CAD build for the part. Positions are in the model's coordinates, mm. A direction names the side the tool comes from. Round coordinates to 2 decimals unless told otherwise and drop trailing zeros. Order: outer loops, then holes, each group sorted by start corner. A loop starts at its lowest first (then second) coordinate and runs counter-clockwise, first axis right, second up. Notation, with made-up numbers: M 42,81.25 L 54,81.25 A20 cw 54,94.25 Z; hole C 62.25,75.5 d6. An arc over 180 degrees is marked long. Answer as a JSON object with one key per item and string values. Group by question number.
Autodesk Inventor part; units mm, degrees
ref_plane "YZ Plane" through (0, 0, 0) normal (1, 0, 0) x (0, 1, 0)
ref_plane "XZ Plane" through (0, 0, 0) normal (0, 1, 0) x (-1, 0, 0)
ref_plane "XY Plane" through (0, 0, 0) normal (0, 0, 1) x (1, 0, 0)
sketch "Sketch1" plane through (0, 0, 0) normal (0, 0, 1) x (1, 0, 0)
  line L0 (0, 4) -> (0, -4)
  line L1 (0, -4) -> (1.25, -4)
  line L2 (1.25, -4) -> (1.5, -3.75)
  line L3 (1.5, -3.75) -> (1.5, 0.9)
  line L4 (1.6, 1) -> (2.5, 1)
  line L5 (2.75, 1.25) -> (2.75, 3.75)
  line L6 (2.5, 4) -> (0, 4)
  arc A0 (1.6, 1) -> (1.5, 0.9) centre (1.6, 0.9) ccw
  line L7 (2.5, 4) -> (2.75, 3.75)
  line L8 (2.5, 1) -> (2.75, 1.25)
  point P0 (0, 0)
  point P1 (2.75, 1)
  point P2 (2.75, 4)
  point P3 (0, 0)
  dimension "d0" = 5.5
  dimension "d1" = 3
  dimension "d3" = 3
  dimension "d4" = 3.2
  dimension "d5" = 135
  dimension "d6" = 0.25
  dimension "d7" = 5
  dimension "d18" = 0.25
revolve "Revolution1" add sketch "Sketch1" angle 360 about axis through (0, 4, 0) along (0, -1, 0)
sketch "Sketch2" plane through (0, 4, 0) normal (0, 1, 0) x (1, 0, 0)
  line L0 (0, -1.4434) -> (-1.25, -0.7217)
  line L1 (-1.25, -0.7217) -> (-1.25, 0.7217)
  line L2 (-1.25, 0.7217) -> (0, 1.4434)
  line L3 (0, 1.4434) -> (1.25, 0.7217)
  line L4 (1.25, 0.7217) -> (1.25, -0.7217)
  line L5 (1.25, -0.7217) -> (0, -1.4434)
  point P0 (0, 0)
  point P1 (0, 0)
  dimension "d11" = 2.5
extrude "Extrusion1" cut sketch "Sketch2" against normal blind 1.5
thread "Thread1"
sketch "Sketch3" plane through (0, 0, 0) normal (1, 0, 0) x (0, 1, 0)
  line L0 (4, 1.4434) -> (4, 0.7217)
  line L1 (4, 1.4434) -> (3.5, 0.9434)
  line L2 (3.5, 0.9434) -> (4, 0.9434)
  line L3 (4, 0.9434) -> (4, 1.4434)
  line L4 (-0.9, 0) -> (5.4, 0)
  point P0 (0, 0)
  dimension "d16" = 0.5
revolve "Revolution2" cut sketch "Sketch3" angle 360 about axis through (0, -10, 0) along (0, 1, 0)
properties part number "48-0350" material "Stainless Steel"
Item 1: Cut at A-A, the plane z = 0. Give the cut face in (x, y).
Item 2: 3-axis set-ups, long thin cutter, end or side, ignore diameter. For faces 1 (the face through (0, -4, 0)), 2 (the face through (-0.616, 3.261, 1.088)): which of +Z, -Z, +X, -X, +Y, -Y reach the whole face in a straight line?
Item 3: Flat gauge pins, fed straight in: pin 1 Ø3 at (x, y) = (-0.5, -3) entering from +Z; pin 2 Ø1.5 at (y, z) = (-1.5, 1.5) entering from -X; pin 3 Ø3 at (y, z) = (2.5, 1.5) entering from -X; pin 4 Ø1.5 at (y, z) = (-2.5, -0.5) entering from +X. Where does each tip first touch, or does it go through?
Item 4: Two-plate mould, pull along Z, no slides. Class faces 3 (the face through (-1.5, -1.39, -0.07)), 4 (the face through (2, 1, 0)), 5 (the face through (0, 2.5, 0)): +Z half, -Z half, draft (parallel to the pull), parting line (faces both ways), or undercut.
Item 5: Drill centre lines: line 1 (Y direction, x = -0.85, z = -1.4); line 2 (X direction, y = 3, z = 0.6); line 3 (Y direction, x = -0.4, z = 1.15). Where is each one in solid material? Low to high. Write a range as [from, to].
Item 6: Cut at B-B, the plane y = -1.75. Give the cut face in (x, z), and give its area (3 significant figures).
Response values:
{
 "1": {"outline": "M -2.75,1.25 L -2.5,1 L -1.6,1 A0.1 cw -1.5,0.9 L -1.5,-3.75 L -1.25,-4 L 1.25,-4 L 1.5,-3.75 L 1.5,0.9 A0.1 cw 1.6,1 L 2.5,1 L 2.75,1.25 L 2.75,3.75 L 2.5,4 L 1.44,4 L 1.25,3.81 L 1.25,2.5 L -1.25,2.5 L -1.25,3.81 L -1.44,4 L -2.5,4 L -2.75,3.75 Z"},
 "2": {"face 1": "+Z, -Z, +X, -X, -Y", "face 2": "+Y"},
 "3": {"pin 1": "z = 1.5", "pin 2": "x = -1.3", "pin 3": "x = -2.75", "pin 4": "x = 1.5"},
 "4": {"face 3": "parting line", "face 4": "draft", "face 5": "undercut"},
 "5": {"line 1": "[1, 4]", "line 2": "[-2.68, -1.25], [1.25, 2.68]", "line 3": "[-4, 2.5]"},
 "6": {"outline": "C 0,0 d3", "area": "7.07 mm^2"}
}
